from build123d import *

# Parameters (mm, degrees)
F0_W      = 25.4
F0_H      = 19.05
F1_DEPTH  = 0.79375
F2_R      = 2.38125
F3_W      = 19.05
F3_H      = 15.875
F4_DEPTH  = 4.9276
F5_W      = 12.7
F5_H      = 1.27
F6_DEPTH  = 0.79375
F7_R      = 1.58749
F8_R      = 1.5875
F9_W      = 12.7
F9_H      = 1.27
F9_W_2    = 15.875
F9_H_2    = 14.2875
F10_DEPTH = 0.79375
F11_R     = 0.79374
F12_R     = 0.79375


# Not quite as in the source:
# - a fillet or chamfer is up to 0.001 mm smaller than in the source, because OpenCascade refuses the exact size
# - ends of sketch curves that miss each other by under 0.0002 mm in the source are joined


with BuildPart() as f1:
    # F0 (on Front) → F1 (new body)
    with BuildSketch(Plane.XZ):
        Rectangle(F0_W, F0_H)
    extrude(amount=F1_DEPTH)

    # F2
    f2_edges = [f1.edges().sort_by_distance(p)[0] for p in [
        (12.7, -0.396875, -9.525),
        (-12.7, -0.396875, -9.525),
    ]]
    fillet(f2_edges, radius=F2_R)

    # F3 (on face) → F4 (cut)
    with BuildSketch(Plane.XZ.offset(0.79375)):
        with Locations((0, 1.5875)):
            Rectangle(F3_W, F3_H)
    extrude(amount=-F4_DEPTH, mode=Mode.SUBTRACT)

    # F5 (on face) → F6 (join)
    with BuildSketch(Plane.XZ.offset(0.79375)):
        Polygon((-15.875, 15.875), (-15.875, 9.525), (-12.7, 9.525), (-9.525, 9.525), (9.525, 9.525), (12.7, 9.525), (15.875, 9.525), (15.875, 15.875), align=None)
        with Locations((0, 12.7)):
            Rectangle(F5_W, F5_H, mode=Mode.SUBTRACT)
    extrude(amount=-F6_DEPTH)

    # F7 (radius 1.5875 in the source; OpenCascade refuses exactly that, so slightly less here)
    f7_edges = [f1.edges().sort_by_distance(p)[0] for p in [
        (-15.875, -0.396875, 15.875),
        (15.875, -0.396875, 15.875),
        (15.875, -0.396875, 9.525),
        (12.7, -0.396875, 9.525),
        (-15.875, -0.396875, 9.525),
        (-12.7, -0.396875, 9.525),
    ]]
    fillet(f7_edges, radius=F7_R)

    # F8
    f8_edges = [f1.edges().sort_by_distance(p)[0] for p in [
        (-9.525, -0.396875, -6.35),
        (9.525, -0.396875, -6.35),
    ]]
    fillet(f8_edges, radius=F8_R)

    # F9 (on face) → F10 (join)
    with BuildSketch(Plane.XZ.offset(0.79375)):
        with BuildLine():
            ThreePointArc((-14.28751, 15.875), (-15.4100349441, 15.4100349441), (-15.875, 14.28751))
            Line((-15.875, 14.28751), (-15.875, 11.11249))
            ThreePointArc((-15.875, 11.11249), (-15.4100349441, 9.9899650559), (-14.28751, 9.525))
            ThreePointArc((-14.28751, 9.525), (-13.1649650559, 9.0600349441), (-12.7, 7.93751))
            Line((-12.7, 7.93751), (-12.7, -7.14375))
            ThreePointArc((-12.7, -7.14375), (-12.0025480227, -8.8275480227), (-10.31875, -9.525))
            Line((-10.31875, -9.525), (10.31875, -9.525))
            ThreePointArc((10.31875, -9.525), (12.0025480227, -8.8275480227), (12.7, -7.14375))
            Line((12.7, -7.14375), (12.7, 7.93751))
            ThreePointArc((12.7, 7.93751), (13.1649650559, 9.0600349441), (14.28749, 9.525))
            ThreePointArc((14.28749, 9.525), (15.4100349441, 9.9899650559), (15.875, 11.11249))
            Line((15.875, 11.11249), (15.875, 14.28751))
            ThreePointArc((15.875, 14.28751), (15.4100349441, 15.4100349441), (14.28751, 15.875))
            Line((14.28751, 15.875), (-14.28751, 15.875))
        make_face()
        with BuildLine():
            Line((-9.525, 9.525), (-7.9375, 9.525))
            Line((-7.9375, 9.525), (7.9375, 9.525))
            Line((7.9375, 9.525), (9.525, 9.525))
            Line((9.525, 9.525), (9.525, -4.7625))
            ThreePointArc((9.525, -4.7625), (9.0600320151, -5.8850320151), (7.9375, -6.35))
            Line((7.9375, -6.35), (-7.9375, -6.35))
            ThreePointArc((-7.9375, -6.35), (-9.0600320151, -5.8850320151), (-9.525, -4.7625))
            Line((-9.525, -4.7625), (-9.525, 9.525))
        make_face(mode=Mode.SUBTRACT)
        with Locations((0, 12.7)):
            Rectangle(F9_W, F9_H, mode=Mode.SUBTRACT)
        with Locations((0, 2.38125)):
            Rectangle(F9_W_2, F9_H_2)
    extrude(amount=-F10_DEPTH)

    # F11 (radius 0.79375 in the source; OpenCascade refuses exactly that, so slightly less here)
    f11_edges = [f1.edges().sort_by_distance(p)[0] for p in [
        (-7.9375, -0.396875, 9.525),
        (-9.525, -0.396875, 9.525),
        (7.9375, -0.396875, 9.525),
        (9.525, -0.396875, 9.525),
    ]]
    fillet(f11_edges, radius=F11_R)

    # F12
    f12_edges = [f1.edges().sort_by_distance(p)[0] for p in [
        (-7.9375, -0.396875, -4.7625),
        (7.9375, -0.396875, -4.7625),
    ]]
    fillet(f12_edges, radius=F12_R)


solid = f1.part
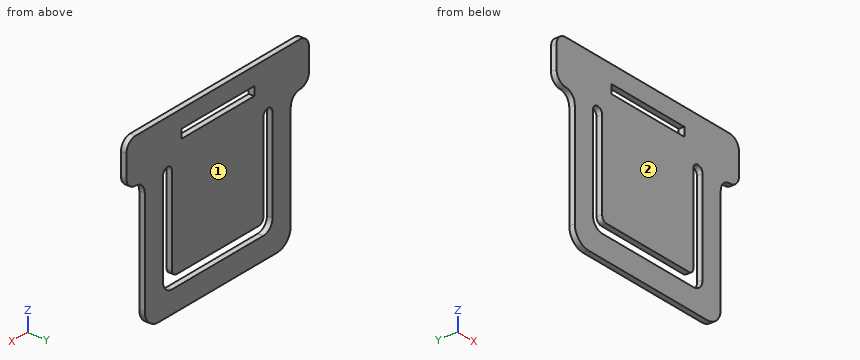
Input: part model. Units: mm. Frame: model coordinates. Face numbers are marked on the shaded views. Coordinates: 2 decimals unless noted, no trailing zeros. Order: outer loops, then holes, each group sorted by start corner. A loop starts at its lowest first (then second) coordinate and runs counter-clockwise, first axis right, second up.
1. Cut plane B-B, the plane z = -0.75. Return loops of the section in (x, y) (1 decimal).
Checked values:
outline: (-12.7, -0.8) - (-9.5, -0.8) - (-9.5, 0) - (-12.7, 0) - close; (-7.9, -0.8) - (7.9, -0.8) - (7.9, 0) - (-7.9, 0) - close; (9.5, -0.8) - (12.7, -0.8) - (12.7, 0) - (9.5, 0) - close
2. Ray query, line 1 along X through (y, z) = (-0.3, 1) (1 decimal); line 2 along X through (y, z) = (-0.25, 13) (3 decimals); line 3 along Z through (x, y) = (-9, -0.25) (3 decimals). Return the intervals inside material, ascending.
Checked values:
line 1: x = -12.7 to -9.5, -7.9 to 7.9, 9.5 to 12.7
line 2: x = -15.875 to -6.35, 6.35 to 15.875
line 3: z = -9.525 to -5.942, 9.478 to 15.875
3. Cut plane A-A, the plane x = -2.5. Count the separate pieces of the cut face and the enclosed holes in it, plus the area to 3 significant figures.
Checked values:
separate pieces: 3
enclosed holes: 0
area: 17.9 mm2
4. Cut plane D-D, the plane x = -12. Return loops of the section in (y, z) (3 decimals), plus the area to 3 significant figures.
Checked values:
outline: (-0.794, -8.83) - (0, -8.83) - (0, 15.875) - (-0.794, 15.875) - close
area: 19.6 mm2
5. Draft query along Y for the marked faces 1 and 2. Return one class per face: +Y half, -Y half, draft (parallel to the pull), parting line (faces both ways), or undercut.
Checked values:
face 1: +Y half
face 2: -Y half
